Autodesk Inventor part; units mm, degrees
ref_plane "YZ Plane" through (0, 0, 0) normal (1, 0, 0) x (0, 1, 0)
ref_plane "XZ Plane" through (0, 0, 0) normal (0, 1, 0) x (-1, 0, 0)
ref_plane "XY Plane" through (0, 0, 0) normal (0, 0, 1) x (1, 0, 0)
sketch "Sketch1" plane through (0, 0, 0) normal (0, 0, 1) x (1, 0, 0)
  line L0 (173.1273, 69.5507) -> (165.6273, 56.5604)
  line L1 (165.6273, 56.5604) -> (163.0292, 58.0604)
  line L2 (163.0292, 58.0604) -> (170.5292, 71.0507)
  line L3 (170.5292, 71.0507) -> (173.1273, 69.5507)
  line L4 (113.6574, 26.5556) -> (98.6574, 26.5556)
  line L5 (98.6574, 26.5556) -> (98.6574, 29.5556)
  line L6 (98.6574, 29.5556) -> (113.6574, 29.5556)
  line L7 (113.6574, 29.5556) -> (113.6574, 26.5556)
  line L8 (46.6875, 142.5507) -> (49.2856, 141.0507)
  line L9 (49.2856, 141.0507) -> (41.7856, 128.0604)
  line L10 (41.7856, 128.0604) -> (39.1875, 129.5604)
  line L11 (39.1875, 129.5604) -> (46.6875, 142.5507)
  line L12 (46.6875, 56.5604) -> (39.1875, 69.5507)
  line L13 (39.1875, 69.5507) -> (41.7856, 71.0507)
  line L14 (41.7856, 71.0507) -> (49.2856, 58.0604)
  line L15 (49.2856, 58.0604) -> (46.6875, 56.5604)
  line L16 (98.6574, 172.5556) -> (113.6574, 172.5556)
  line L17 (113.6574, 172.5556) -> (113.6574, 169.5556)
  line L18 (113.6574, 169.5556) -> (98.6574, 169.5556)
  line L19 (98.6574, 169.5556) -> (98.6574, 172.5556)
  line L20 (165.6273, 142.5507) -> (173.1273, 129.5604)
  line L21 (173.1273, 129.5604) -> (170.5292, 128.0604)
  line L22 (170.5292, 128.0604) -> (163.0292, 141.0507)
  line L23 (163.0292, 141.0507) -> (165.6273, 142.5507)
  line L24 (290, 0) -> (290, 200)
  line L25 (290, 200) -> (0, 200)
  line L26 (0, 200) -> (0, 0)
  line L27 (0, 0) -> (290, 0)
  circle A0 centre (281.9574, 20.463) radius 2.5
  circle A1 centre (49.9574, 20.463) radius 2.5
  circle A2 centre (281.9574, 180.463) radius 2.5
  circle A3 centre (49.9574, 180.463) radius 2.5
  circle A4 centre (242.3574, 20.463) radius 2.5
  circle A5 centre (17.5, 20) radius 2.5
  circle A6 centre (17.5, 180) radius 2.5
  circle A7 centre (242.3574, 180.463) radius 2.5
  line L28 (0, 0) -> (0, 10)
  line L29 (0, 10) -> (0, 15)
  line L30 (0, 200) -> (0, 185)
  line L31 (0, 185) -> (60, 185)
  line L32 (60, 185) -> (60, 175)
  line L33 (60, 175) -> (0, 175)
  line L34 (0, 15) -> (70, 15)
  line L35 (70, 15) -> (70, 25)
  line L36 (70, 25) -> (0, 25)
  line L37 (60, 185) -> (70, 185)
  line L38 (70, 185) -> (70, 175)
  line L39 (70, 175) -> (60, 175)
  line L40 (281.9574, 20.463) -> (242.3574, 20.463)
  line L41 (242.3574, 20.463) -> (130.1488, 20.463)
  circle A8 centre (182.3574, 20.463) radius 2.5
  circle A9 centre (142.7574, 20.463) radius 2.5
  line L42 (0, 100) -> (290, 100)
  line L43 (242.3574, 179.537) -> (130.1488, 179.537)
  circle A10 centre (182.3574, 179.537) radius 2.5
  circle A11 centre (142.7574, 179.537) radius 2.5
  circle A12 centre (17.5, 59.6) radius 2.5
  circle A13 centre (17.5, 140.4) radius 2.5
  line L44 (40, 35.2) -> (86.2, 35.2)
  line L45 (86.2, 35.2) -> (86.2, 15)
  line L46 (86.2, 15) -> (40, 15)
  line L47 (40, 15) -> (40, 35.2)
  line L48 (40, 164.8) -> (86.2, 164.8)
  line L49 (86.2, 164.8) -> (86.2, 185)
  line L50 (86.2, 185) -> (40, 185)
  line L51 (40, 185) -> (40, 164.8)
  line L52 (17.5, 20) -> (17.5, 180)
  line L53 (55, 50) -> (66, 50)
  line L54 (66, 50) -> (66, 82)
  line L55 (66, 82) -> (55, 82)
  line L56 (55, 82) -> (55, 50)
  circle A14 centre (60.5, 52.5) radius 1.5
  circle A15 centre (60.5, 79.5) radius 1.5
  line L57 (54.4, 54.75) -> (66.6, 54.75)
  line L58 (66.6, 54.75) -> (66.6, 77.25)
  line L59 (66.6, 77.25) -> (54.4, 77.25)
  line L60 (54.4, 77.25) -> (54.4, 54.75)
  line L61 (55, 150) -> (66, 150)
  line L62 (66, 150) -> (66, 118)
  line L63 (66, 118) -> (55, 118)
  line L64 (55, 118) -> (55, 150)
  circle A16 centre (60.5, 147.5) radius 1.5
  circle A17 centre (60.5, 120.5) radius 1.5
  line L65 (54.4, 145.25) -> (66.6, 145.25)
  line L66 (66.6, 145.25) -> (66.6, 122.75)
  line L67 (66.6, 122.75) -> (54.4, 122.75)
  line L68 (54.4, 122.75) -> (54.4, 145.25)
  point P0 (66.6, 66)
  point P1 (66, 66)
  point P2 (60.5, 54.75)
  point P3 (60.5, 50)
  point P4 (66.6, 134)
  point P5 (66, 134)
  point P6 (60.5, 145.25)
  point P7 (60.5, 150)
  dimension "d2" = 10
  dimension "d3" = 5
  dimension "d6" = 15
  dimension "d7" = 60
  dimension "d8" = 10
  dimension "d9" = 70
  dimension "d10" = 10
  dimension "d11" = 10
  dimension "d12" = 10
  dimension "d13" = 5
  dimension "d14" = 5
  dimension "d15" = 39.6
  dimension "d16" = 39.6
  dimension "d17" = 60
  dimension "d18" = 8.0426
  dimension "d19" = 39.6
  dimension "d20" = 20.2
  dimension "d21" = 46.2
  dimension "d22" = 15
  dimension "d23" = 40
  dimension "d24" = 17.5
  dimension "d25" = 5
  dimension "d26" = 5
  dimension "d27" = 20
  dimension "d28" = 20
  dimension "d29" = 39.6
  dimension "d30" = 55
  dimension "d31" = 50
  dimension "d32" = 11
  dimension "d33" = 32
  dimension "d34" = 3
  dimension "d35" = 3
  dimension "d36" = 2.5
  dimension "d37" = 2.5
  dimension "d38" = 22.5
  dimension "d39" = 12.2
extrude "Extrusion1" add sketch "Sketch1" along normal blind 3 contours L27 L26 L34 L46 L45 L44 L47 L36 L52 A12 L42 L24 | L42 L52 A13 L33 L51 L48 L49 L50 L37 L31 L26 L25 L24 | L52 A12 L36 L26 L42 | L42 L26 L33 L52 A13 | L26 L36 L47 L34 | L31 L51 L33 L26 | A9 L41 | L41 A9 | A8 L41 | L41 A8 | A11 L43 | L43 A11 | A10 L43 | L43 A10 | L56 L57 L54 L53 | L56 L55 L54 L59 | L61 L62 L65 L64 | L67 L62 L63 L64
properties material "MDF Medium Density Fiberboard"
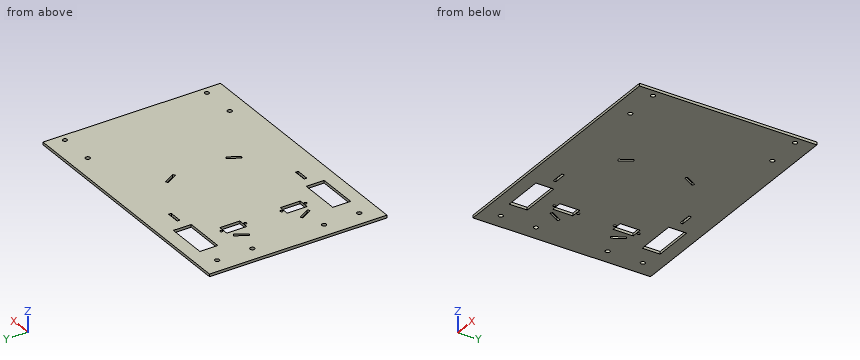
The model under review builds one solid part; all positions refer to its coordinate system, in mm. Give positions to 0.01 mm unless a question says otherwise; leave off trailing zeros. Write each loop counter-clockwise with the first axis right and the second up, starting at its lowest first coordinate (ties: lowest second). Pieces come first, ordered by that corner, then holes.
(1) To check wall thickness, follow L1, parallel to Y at x = 17.5, z = 0.85; L2, parallel to Y at x = 50, z = 0.2; L3, parallel to X at y = 175, z = 1.75. State the ranges of each line that lie inside material, in increasing order.
(2) Consider section B-B, the plane z = 1.3. Give the number of separate pieces and of enclosed holes in the cut face, and give its area (3 significant figures).
(3) Consider section A-A, the plane y = 74. Give the boundary of the cut face in (x, z).
(4) For P1, Ø1.5, axis at y = 71, z = 1.5, coming from the -X side, flat-tipped, find the tip position at first contact; note if it passes through.
Returned:
1. L1: y = 0 to 17.5, 22.5 to 57.1, 62.1 to 137.9, 142.9 to 177.5, 182.5 to 200
1. L2: y = 0 to 15, 35.2 to 164.8, 185 to 200
1. L3: x = 0 to 40, 86.2 to 290
2. separate pieces: 1
2. enclosed holes: 22
2. area: 55,100 mm2
3. outline: (0, 0) - (54.4, 0) - (54.4, 3) - (0, 3) - close; (66.6, 0) - (290, 0) - (290, 3) - (66.6, 3) - close
4. P1: stops at x = 0
